CAD build for the part. Positions are in the model's coordinates, mm. A direction names the side the tool comes from. Round coordinates to 2 decimals unless told otherwise and drop trailing zeros. Write each loop counter-clockwise with the first axis right and the second up, starting at its lowest first coordinate (ties: lowest second). Pieces come first, ordered by that corner, then holes. Notation, with made-up numbers: (39.5, 58.25) - (55.5, 58.25) arc R22 ccw to (55.5, 94.25) - close; hole circle Ø1 at (12, 80.5). An arc over 180 degrees is marked (long way). Answer in a Markdown table with one row per item.
```python
from build123d import *

# Parameters (mm, degrees)
SKETCH_1_R      = 2.6
EXTRUDE_1_DEPTH = 5
FILLET_1_R      = 4


with BuildPart() as part:
    # 草图1 → 凸台-拉伸1 (new body)
    with BuildSketch(Plane(origin=(0, 0, 0), x_dir=(1, 0, 0), z_dir=(0, 1, 0))):
        Polygon((-40, 0), (-25.5, 0), (-25.5, -50), (25.5, -50), (25.5, 0), (40, 0), (40, 30), (-40, 30), align=None)
        with Locations(Location((-32, 15, 0), (0, 0, 270))):
            Circle(SKETCH_1_R, mode=Mode.SUBTRACT)
        with Locations(Location((32, 15, 0), (0, 0, 90))):
            Circle(SKETCH_1_R, mode=Mode.SUBTRACT)
        with BuildLine():
            Line((18.75, 0), (18.75, -40))
            ThreePointArc((18.75, -40), (16.5, -42.25), (14.25, -40))
            Line((14.25, -40), (14.25, 0))
            ThreePointArc((14.25, 0), (16.5, 2.25), (18.75, 0))
        make_face(mode=Mode.SUBTRACT)
        with BuildLine():
            Line((-18.75, 0), (-18.75, -40))
            ThreePointArc((-18.75, -40), (-16.5, -42.25), (-14.25, -40))
            Line((-14.25, -40), (-14.25, 0))
            ThreePointArc((-14.25, 0), (-16.5, 2.25), (-18.75, 0))
        make_face(mode=Mode.SUBTRACT)
    extrude(amount=EXTRUDE_1_DEPTH)

    # 圆角1
    fillet_1_edges = [part.edges().sort_by_distance(p)[0] for p in [
        (-40, 2.5, -30),
        (40, 2.5, -30),
        (40, 2.5, 0),
        (25.5, 2.5, 0),
        (25.5, 2.5, 50),
        (-25.5, 2.5, 50),
        (-25.5, 2.5, 0),
        (-40, 2.5, 0),
    ]]
    fillet(fillet_1_edges, radius=FILLET_1_R)


solid = part.part
```
Q1. Saw through at A-A on z = 21. List the corners of the cut face in (x, y), then the cut area to 3 significant figures.
Computed:
| item | result |
|---|---|
| outline | (-25.5, 0) - (-18.75, 0) - (-18.75, 5) - (-25.5, 5) - close; (-14.25, 0) - (14.25, 0) - (14.25, 5) - (-14.25, 5) - close; (18.75, 0) - (25.5, 0) - (25.5, 5) - (18.75, 5) - close |
| area | 210 mm2 |
Q2. Pull direction Z, two halves, no side cores. Call faces 1 (the flat face through (-40, 2, -15)), 2 (the cylindrical face through (-24.359, 2.535, 48.797)), 3 (the flat face through (-14.25, 2, 20)): released by +Z, released by -Z, zero draft, split by the parting line, or undercut.
Computed:
| item | result |
|---|---|
| face 1 | zero draft |
| face 2 | released by +Z |
| face 3 | undercut |
Q3. 3-axis set-ups, long thin cutter, end or side, ignore diameter. For faces 4 (the flat face through (-1, 0, 1)), 5 (the flat face through (33, 2, 0)), 6 (the flat face through (-33, 2, 0)), 7 (the cylindrical face through (16.45, 2.46, -2.25)): which of +Z, -Z, +X, -X, +Y, -Y reach the whole face in a straight line?
Computed:
| item | result |
|---|---|
| face 4 | +Z, -Z, +X, -X, -Y |
| face 5 | +Z, +X, +Y, -Y |
| face 6 | +Z, -X, +Y, -Y |
| face 7 | +Y, -Y |
Q4. Drill centre lines: line 1 (X direction, y = 1.15, z = 10); line 2 (X direction, y = 1.8, z = -15); line 3 (Z direction, x = 32, y = 3.8). Where is each one in solid material? Low to high.
Computed:
| item | result |
|---|---|
| line 1 | x = -25.5 to -18.75, -14.25 to 14.25, 18.75 to 25.5 |
| line 2 | x = -40 to -34.6, -29.4 to 29.4, 34.6 to 40 |
| line 3 | z = -30 to -17.6, -12.4 to 0 |
Q5. Saw through at C-C on y = 4. List the corners of the cut face in (x, z).
Computed:
| item | result |
|---|---|
| outline | (-40, -26) arc R4 ccw to (-36, -30) - (36, -30) arc R4 ccw to (40, -26) - (40, -4) arc R4 ccw to (36, 0) - (29.5, 0) arc R4 cw to (25.5, 4) - (25.5, 46) arc R4 ccw to (21.5, 50) - (-21.5, 50) arc R4 ccw to (-25.5, 46) - (-25.5, 4) arc R4 cw to (-29.5, 0) - (-36, 0) arc R4 ccw to (-40, -4) - close; hole circle Ø5.2 at (-32, -15); hole (-18.75, 0) arc R2.25 ccw to (-14.25, 0) - (-14.25, 40) arc R2.25 ccw to (-18.75, 40) - close; hole (14.25, 0) arc R2.25 ccw to (18.75, 0) - (18.75, 40) arc R2.25 ccw to (14.25, 40) - close; hole circle Ø5.2 at (32, -15) |
Q6. Flat gauge pins, fed straight in: pin 1 (1.5 mm diameter, centred on y = 2, z = 16, fed in from +X); pin 2 (2 mm diameter, centred on x = -25, y = 3, fed in from +Z); pin 3 (1.5 mm diameter, centred on y = 3, z = 33, fed in from -X); pin 4 (8.5 mm diameter, centred on x = -32, z = -15, fed in from +Y). Where does each tip first touch, or does it go through?
Computed:
| item | result |
|---|---|
| pin 1 | stops at x = 25.5 |
| pin 2 | stops at z = 49.12 |
| pin 3 | stops at x = -25.5 |
| pin 4 | stops at y = 5 |
Q7. Saw through at D-D on z = -15. List the corners of the cut face in (x, y).
Computed:
| item | result |
|---|---|
| outline | (-40, 0) - (-34.6, 0) - (-34.6, 5) - (-40, 5) - close; (-29.4, 0) - (29.4, 0) - (29.4, 5) - (-29.4, 5) - close; (34.6, 0) - (40, 0) - (40, 5) - (34.6, 5) - close |
Q8. Saw through at B-B on x = -32. List the corners of the cut face in (y, z), then the cut area to 3 significant figures.
Computed:
| item | result |
|---|---|
| outline | (0, -30) - (5, -30) - (5, -17.6) - (0, -17.6) - close; (0, -12.4) - (5, -12.4) - (5, 0) - (0, 0) - close |
| area | 124 mm2 |
